Build history of the part. All positions in model axes, mm. A direction names the side the tool comes from. Give positions to 0.01 mm unless a question says otherwise; leave off trailing zeros. Loops run counter-clockwise (first coordinate to the right, second up) from the corner with the lowest first, then second, coordinate; pieces in that order, holes last. Notation, with made-up numbers: M 26.25,-8.5 L 63.25,-8.5 A11 ccw 63.25,8.5 Z; hole C -21,13.5 d11. An arc over 180 degrees is marked long. Put each result on its own line as item: value.
```python
from build123d import *

# Parameters (mm, degrees)
BOX019_W     = 1.2
BOX019_H     = 3
BOX019_DEPTH = 3.4
BOX020_W     = 1.2
BOX020_H     = 3
BOX020_DEPTH = 3.4
BOX018_W     = 9.8
BOX018_H     = 4.3
BOX018_DEPTH = 5
BOX017_W     = 3
BOX017_H     = 1
BOX017_DEPTH = 5


with BuildPart() as obj1:
    # Box019 → Box019 (new body)
    with BuildSketch(Plane(origin=(-3.45, -1.5, 2.45), x_dir=(1, 0, 0), z_dir=(0, 0, 1))):
        with Locations((0.6, 1.5)):
            Rectangle(BOX019_W, BOX019_H)
    extrude(amount=BOX019_DEPTH)


with BuildPart() as obj2:
    # Box020 → Box020 (new body)
    with BuildSketch(Plane(origin=(2.25, -1.5, 2.45), x_dir=(1, 0, 0), z_dir=(0, 0, 1))):
        with Locations((0.6, 1.5)):
            Rectangle(BOX020_W, BOX020_H)
    extrude(amount=BOX020_DEPTH)

    # Fusion002: union obj1
    add(obj1.part)


with BuildPart() as obj3:
    # Box018 → Box018 (new body)
    with BuildSketch(Plane(origin=(-4.9, -2.15, 0.85), x_dir=(1, 0, 0), z_dir=(0, 0, 1))):
        with Locations((4.9, 2.15)):
            Rectangle(BOX018_W, BOX018_H)
    extrude(amount=BOX018_DEPTH)


with BuildPart() as obj4:
    # Box017 → Box017 (new body)
    with BuildSketch(Plane(origin=(-1.5, -3.15, 0.85), x_dir=(1, 0, 0), z_dir=(0, 0, 1))):
        with Locations((1.5, 0.5)):
            Rectangle(BOX017_W, BOX017_H)
    extrude(amount=BOX017_DEPTH)

    # Fusion003: union obj3
    add(obj3.part)

    # Cut002: cut obj2
    add(obj2.part, mode=Mode.SUBTRACT)


solid = obj4.part
```
Q1. Slice it at B-B (x = -3). List the corners of the cut face in (y, z).
Here are the results:
outline: M -2.15,0.85 L 2.15,0.85 L 2.15,5.85 L 1.5,5.85 L 1.5,2.45 L -1.5,2.45 L -1.5,5.85 L -2.15,5.85 Z
Q2. Slice it at C-C (z = 1.55). List the corners of the cut face in (x, y).
Here are the results:
outline: M -4.9,-2.15 L -1.5,-2.15 L -1.5,-3.15 L 1.5,-3.15 L 1.5,-2.15 L 4.9,-2.15 L 4.9,2.15 L -4.9,2.15 Z
Q3. Slice it at A-A (z = 4.75). List the corners of the cut face in (x, y).
Here are the results:
outline: M -4.9,-2.15 L -1.5,-2.15 L -1.5,-3.15 L 1.5,-3.15 L 1.5,-2.15 L 4.9,-2.15 L 4.9,2.15 L -4.9,2.15 Z; hole M -3.45,-1.5 L -2.25,-1.5 L -2.25,1.5 L -3.45,1.5 Z; hole M 2.25,-1.5 L 3.45,-1.5 L 3.45,1.5 L 2.25,1.5 Z
Q4. Mould opens along Y. For faces 1 (the flat face through (-3.45, 0, 4)), 2 (the flat face through (0, 2.15, 3)), 3 (the flat face through (3, -2.15, 3)), 4 (the flat face through (-1.5, -2.7, 3.3)) say: pulls with the +Y half, pulls with the -Y half, needs draft (parallel to the pull), parting line crosses it, or undercut.
Here are the results:
face 1: undercut
face 2: pulls with the +Y half
face 3: pulls with the -Y half
face 4: needs draft
Q5. Probe line 1 (X direction, y = 1.4, z = 4.9); line 2 (Y direction, x = 3, z = 3.95); line 3 (Z direction, x = -2.5, y = -0.65). List the from-to ranges inside material, lowest first. Write a range as from..to.
Here are the results:
line 1: -4.9..-3.45, -2.25..2.25, 3.45..4.9
line 2: -2.15..-1.5, 1.5..2.15
line 3: 0.85..2.45
Q6. Slice it at D-D (y = -1.15). List the corners of the cut face in (x, z).
Here are the results:
outline: M -4.9,0.85 L 4.9,0.85 L 4.9,5.85 L 3.45,5.85 L 3.45,2.45 L 2.25,2.45 L 2.25,5.85 L -2.25,5.85 L -2.25,2.45 L -3.45,2.45 L -3.45,5.85 L -4.9,5.85 Z
Q7. Drop flat-ended pins along their axis: pin 1 Ø2 at (x, y) = (-3, 1) entering from +Z; pin 2 Ø0.5 at (y, z) = (-3, 3) entering from -X; pin 3 Ø1 at (x, z) = (3, 3.5) entering from -Y. Give the stop position or say it passes through.
Here are the results:
pin 1: z = 5.85
pin 2: x = -1.5
pin 3: y = -2.15
Q8. Tool access for faces 5 (the flat face through (3, -1.5, 4)), 6 (the flat face through (1.5, -2.7, 3.3)), 7 (the flat face through (4.9, 0, 3)), 8 (the flat face through (0, 0, 5.85)), 9 (the flat face through (-3, -2.15, 3)): list every direction of +Z, -Z, +X, -X, +Y, -Y with a clear straight run to the whole face (end or side of a thin tool).
Here are the results:
face 5: +Z
face 6: +Z, -Z, +X, -Y
face 7: +Z, -Z, +X, +Y, -Y
face 8: +Z, +X, -X, +Y, -Y
face 9: +Z, -Z, -X, -Y
